```python
from build123d import *

# Parameters (mm, degrees)
F0_W     = 435
F0_H     = 332
F1_DEPTH = 26
F2_W     = 399.4
F2_H     = 307.5
F3_DEPTH = 0.5
F4_W     = 290
F4_H     = 190
F5_DEPTH = 32
F6_W     = 45.65622
F6_H     = 10.88232
F7_DEPTH = 5
F8_W     = 131.441295
F8_H     = 230.077163
F9_DEPTH = 30


with BuildPart() as f1:
    # F0 (on Top) → F1 (new body)
    with BuildSketch(Plane.XY):
        Rectangle(F0_W, F0_H)
    extrude(amount=F1_DEPTH)

    # F2 (on face) → F3 (cut)
    with BuildSketch(Plane.XY.offset(26)):
        with Locations((-7.2, -2.75)):
            Rectangle(F2_W, F2_H)
    extrude(amount=-F3_DEPTH, mode=Mode.SUBTRACT)

    # F4 (on face) → F5 (join)
    with BuildSketch(Plane.XY):
        with Locations((-22.5, 9)):
            Rectangle(F4_W, F4_H)
    extrude(amount=-F5_DEPTH)

    # F6 (on face) → F7 (cut)
    with BuildSketch(Plane(origin=(0, 104, 0), x_dir=(-1, 0, 0), z_dir=(0, 1, 0))):
        with Locations((45.32811, -15.279424)):
            Rectangle(F6_W, F6_H)
    extrude(amount=-F7_DEPTH, mode=Mode.SUBTRACT)

    # F8 (on face) → F9 (cut)
    with BuildSketch(Plane.XY.offset(26)):
        with Locations((-68.291783, -5.109631)):
            Rectangle(F8_W, F8_H)
    extrude(amount=-F9_DEPTH, mode=Mode.SUBTRACT)


solid = f1.part
```
Model file for the job. Use its own axes, mm. A direction names the side the tool comes from. Round coordinates to 2 decimals unless told otherwise and drop trailing zeros. Loops run counter-clockwise (first coordinate to the right, second up) from the corner with the lowest first, then second, coordinate; pieces in that order, holes last. Notation, with made-up numbers: M 57.5,63.5 L 115.5,63.5 A29 cw 115.5,95.5 Z; hole C 47,-18.75 d7. An arc over 180 degrees is marked long. Put each result on its own line as item: value. Start each with the question number.
Item 1: Cut at D-D (x = 62.5). List the corners of the cut face in (y, z).
Item 2: Cut at B-B (x = -101.5). List the corners of the cut face in (y, z).
Item 3: Drill centre lines: line 1 along X through (y, z) = (61.5, 4.5); line 2 along Y through (x, z) = (-23.5, 9); line 3 along X through (y, z) = (78, -27). Where is each one in solid material? Low to high.
Item 4: Mould opens along Y. For faces 5 (the face through (122.5, 8, -16)), 6 (the face through (34, -1, 25.5)), 7 (the face through (-25, -86, -16)) say: released by +Y, released by -Y, zero draft, split by the parting line, or undercut.
Item 5: Drop flat-ended pins along their axis: P1, Ø3, axis at x = 8.5, y = -96.5, coming from the -Z side; P2, Ø2, axis at x = 62, y = 69.5, coming from the +Z side; P3, Ø9.5, axis at y = -38, z = -8, coming from the +X side. Give the stop position or say it passes through.
Item 6: Cut at A-A (y = -93.5). List the corners of the cut face in (x, z), then the cut area to 3 significant figures.
Item 7: 3-axis set-ups, long thin cutter, end or side, ignore diameter. For faces 1 (the face through (-25, 104, -23)), 2 (the face through (-167.5, 8, -16)), 3 (the face through (-69, -120.148, 13)), 4 (the face through (-134.012, -7, 11)): which of +Z, -Z, +X, -X, +Y, -Y reach the whole face in a straight line?
Item 8: Cut at C-C (z = 11.5). List the corners of the cut face in (x, y), then the cut area to 3 significant figures.
Answer block:
1. outline: M -166,0 L -86,0 L -86,-32 L 104,-32 L 104,0 L 166,0 L 166,26 L 151,26 L 151,25.5 L -156.5,25.5 L -156.5,26 L -166,26 Z
2. outline: M -166,0 L -120.15,0 L -120.15,25.5 L -156.5,25.5 L -156.5,26 L -166,26 Z; M -86,-32 L 104,-32 L 104,-4 L -86,-4 Z; M 109.93,0 L 166,0 L 166,26 L 151,26 L 151,25.5 L 109.93,25.5 Z
3. line 1: -217.5 to -134.01, -2.57 to 217.5
3. line 2: -166 to -120.15, 109.93 to 166
3. line 3: -167.5 to 122.5
4. face 5: zero draft
4. face 6: undercut
4. face 7: released by -Y
5. P1: z = 0
5. P2: z = 25.5
5. P3: x = 122.5
6. outline: M -217.5,0 L -134.01,0 L -134.01,25.5 L -206.9,25.5 L -206.9,26 L -217.5,26 Z; M -2.57,0 L 217.5,0 L 217.5,26 L 192.5,26 L 192.5,25.5 L -2.57,25.5 Z
6. area: 7,760 mm2
7. face 1: -Z, +X, -X, +Y
7. face 2: -Z, -X, +Y, -Y
7. face 3: +Z, -Z
7. face 4: +Z
8. outline: M -217.5,-166 L 217.5,-166 L 217.5,166 L -217.5,166 Z; hole M -134.01,-120.15 L -2.57,-120.15 L -2.57,109.93 L -134.01,109.93 Z
8. area: 114,000 mm2
